Check sheet for the modelled part. Datum: model origin and axes. Units: mm. Give positions to 0.01 mm unless a question says otherwise; leave off trailing zeros. Order: outer loops, then holes, each group sorted by start corner. A loop starts at its lowest first (then second) coordinate and runs counter-clockwise, first axis right, second up. Notation, with made-up numbers: (-30.75, 69.5) -> (-1.75, 69.5) arc R28 ccw to (-1.75, 101.5) -> close; hole circle Ø3 at (6.25, 6.25). An arc over 180 degrees is marked (long way). Write each question's results on one line, items separated by ' | '.
Autodesk Inventor part; units mm, degrees
ref_plane "YZ Plane" through (0, 0, 0) normal (1, 0, 0) x (0, 1, 0)
ref_plane "XZ Plane" through (0, 0, 0) normal (0, 1, 0) x (-1, 0, 0)
ref_plane "XY Plane" through (0, 0, 0) normal (0, 0, 1) x (1, 0, 0)
sketch "Sketch1" plane through (0, 0, 0) normal (0, 0, 1) x (1, 0, 0)
  line L0 (-9.525, -125) -> (9.525, -125)
  line L1 (9.525, -125) -> (9.525, 125)
  line L2 (9.525, 125) -> (-9.525, 125)
  line L3 (-9.525, 125) -> (-9.525, -125)
  point P0 (0, 0)
  point P1 (0, -125)
  point P2 (9.525, 0)
  dimension "d0" = 19.05
  dimension "d1" = 250
extrude "Extrusion1" add sketch "Sketch1" along normal blind 0.25
sketch "Sketch3" plane through (0, 0, 0.25) normal (0, 0, 1) x (1, 0, 0)
  line L0 (-9.525, 125) -> (-9.525, -125)
  line L1 (9.525, -125) -> (9.525, 125)
  line L2 (9.525, -125) -> (9.525, -122.36)
  line L3 (-9.525, -122.36) -> (-9.525, -125)
  line L4 (0, -125) -> (-4, -125) construction
  line L5 (-4, -125) -> (-4, -121.5) construction
  point P0 (0, 0)
  dimension "d18" = 4
  dimension "d19" = 3.5
hole "Hole2" at (-4, -121.5, 0.25) direction (0, 0, -1) diameter 3 end through all
mirror "Mirror1" about plane through (0, 0, 0) normal (1, 0, 0) of "Hole2"
sketch "Sketch4" plane through (0, 0, 0.25) normal (0, 0, 1) x (1, 0, 0)
  line L0 (-9.525, 125) -> (-9.525, -125)
  line L1 (9.525, -125) -> (9.525, 125)
  line L2 (-9.525, -125) -> (9.525, -125)
  line L3 (9.525, -125) -> (9.525, 46.45)
  line L4 (9.525, 46.45) -> (-9.525, 46.45)
  line L5 (-9.525, 46.45) -> (-9.525, -125)
  point P0 (0, 0)
  dimension "d27" = 171.45
extrude "Extrusion2" cut sketch "Sketch4" against normal blind 10 keep common part
properties part number "tape" material "Stainless Steel"
1. Section check A-A on y = -121.5. Record the cut outline in (x, z) (3 decimals), then the cut area to 3 significant figures.
Verdict:
outline: (-9.525, 0) -> (-5.5, 0) -> (-5.5, 0.25) -> (-9.525, 0.25) -> close; (-2.5, 0) -> (2.5, 0) -> (2.5, 0.25) -> (-2.5, 0.25) -> close; (5.5, 0) -> (9.525, 0) -> (9.525, 0.25) -> (5.5, 0.25) -> close | area: 3.26 mm^2
2. Material ranges on probe 1 along X at (y, z) = (-121.5, 0.15) (3 decimals); probe 2 along Y at (x, z) = (4, 0.2); probe 3 along Y at (x, z) = (5, 0.1), recorded low to high. Write a range as from..to.
Verdict:
probe 1: x = -9.525..-5.5, -2.5..2.5, 5.5..9.525 | probe 2: y = -125..-123, -120..46.45 | probe 3: y = -125..-122.62, -120.38..46.45
3. Section check B-B on x = -4. Record the cut outline in (y, z), then the cut area to 3 significant figures.
Verdict:
outline: (-125, 0) -> (-123, 0) -> (-123, 0.25) -> (-125, 0.25) -> close; (-120, 0) -> (46.45, 0) -> (46.45, 0.25) -> (-120, 0.25) -> close | area: 42.1 mm^2
